Autodesk Inventor part; units mm, degrees
ref_plane "YZ Plane" through (0, 0, 0) normal (1, 0, 0) x (0, 1, 0)
ref_plane "XZ Plane" through (0, 0, 0) normal (0, 1, 0) x (-1, 0, 0)
ref_plane "XY Plane" through (0, 0, 0) normal (0, 0, 1) x (1, 0, 0)
sketch "Sketch1" plane through (0, 0, 0) normal (1, 0, 0) x (0, 1, 0)
  circle A0 centre (0, 0) radius 152.4
  line L0 (-76.2507, 131.953) -> (76.2507, 131.953)
  line L1 (76.2507, 131.953) -> (76.2507, -131.953)
  line L2 (76.2507, -131.953) -> (-76.2507, -131.953)
  line L3 (-76.2507, -131.953) -> (-76.2507, 131.953)
  line L4 (-76.2507, 131.953) -> (76.2507, -131.953) construction
  line L5 (76.2507, 131.953) -> (-76.2507, -131.953) construction
  line L6 (-76.2507, 131.953) -> (-88.9591, 153.9452)
  line L7 (-76.2507, -131.953) -> (-88.9591, -153.9452)
  arc A1 (-88.9591, 153.9452) -> (-88.9591, -153.9452) centre (0, 0) ccw
  line L8 (-88.9591, 153.9452) -> (-177.8, 153.9452)
  line L9 (-177.8, 153.9452) -> (-177.8, -354.0548)
  line L10 (-177.8, -354.0548) -> (0, -354.0548)
  line L11 (0, -354.0548) -> (0, -430.2548)
  line L12 (0, -430.2548) -> (-127, -430.2548)
  line L13 (-127, -430.2548) -> (-127, -354.0548)
  line L14 (-127, -430.2548) -> (-177.8, -430.2548)
  line L15 (-177.8, -430.2548) -> (-177.8, -354.0548)
  line L16 (0, -354.0548) -> (12.7, -354.0548)
  line L17 (12.7, -354.0548) -> (-150.4905, -94.6861)
  line L18 (12.7, -354.0548) -> (34.1986, -340.5282)
  line L19 (34.1986, -340.5282) -> (-128.9918, -81.1595)
  line L20 (12.7, -354.0548) -> (60.6438, -430.2548)
  line L21 (60.6438, -430.2548) -> (82.1424, -416.7282)
  line L22 (82.1424, -416.7282) -> (34.1986, -340.5282)
  line L23 (-177.8, 0) -> (127, 0)
  circle A2 centre (127, 0) radius 304.8
  line L24 (-82.6049, 142.9491) -> (-121.1364, 92.4756)
  line L25 (0, -430.2548) -> (0, -455.6548)
  line L26 (0, -455.6548) -> (235.9429, -455.6548)
  line L27 (82.1424, -416.7282) -> (106.6344, -455.6548)
  line L28 (106.6344, -455.6548) -> (85.1357, -469.1814)
  line L29 (85.1357, -469.1814) -> (60.6438, -430.2548)
  line L30 (95.885, -462.4181) -> (91.6297, -455.6548)
  line L31 (91.6297, -455.6548) -> (98.393, -466.4042)
  line L32 (98.393, -466.4042) -> (120.7006, -452.3686)
  line L33 (106.6344, -455.6548) -> (109.1423, -459.6409)
  line L34 (98.393, -466.4042) -> (67.8539, -485.6188)
  line L35 (85.1357, -469.1814) -> (87.6437, -473.1674)
  line L36 (109.1423, -459.6409) -> (87.6437, -473.1674)
  arc A3 (-88.9591, 153.9452) -> (-150.4905, -94.6861) centre (0, 0) ccw
  line L37 (-128.9918, -81.1595) -> (109.1423, -459.6409)
  line L38 (-150.4905, -94.6861) -> (87.6437, -473.1674)
  line L39 (87.6437, -473.1674) -> (109.1423, -459.6409)
  dimension "d5" = 304.8
  dimension "d6" = 263.906
  dimension "d7" = 25.4
  dimension "d8" = 25.4
  dimension "d9" = 508
  dimension "d10" = 76.2
  dimension "d11" = 127
  dimension "d12" = 12.7
  dimension "d13" = 25.4
  dimension "d14" = 25.4
  dimension "d15" = 304.8
  dimension "d16" = 25.4
  dimension "d17" = 12.7
extrude "Extrusion1" add sketch "Sketch1" along normal blind 6.35 contours A0 L23 A1 L6 L24 | L19 L7 A1 L23 A0 | L19 A2 L17 A1 L7 | L19 L18 L17 A2 | L22 L21 L20 L18 | L27 L26 L29 L21 | L28 L30 L26 | L33 L32 L31 L28 | L26 L30 L28 L29 | L31 L34 L35 L28
sketch "Sketch2" plane through (6.35, 0, 0) normal (1, 0, 0) x (0, 0, -1)
  line L0 (473.1674, 87.6437) -> (459.6409, 109.1423)
  line L1 (-142.9491, -82.6049) -> (-153.9452, -88.9591)
  line L2 (466.4042, 98.393) -> (455.4081, 92.0388)
  circle A0 centre (455.4081, 92.0388) radius 3.175
  dimension "d20" = 12.7
  dimension "d21" = 6.35
extrude "Extrusion2" cut sketch "Sketch2" against normal blind 25.4
sketch "Sketch3" plane through (6.35, 109.1423, -459.6409) normal (0, 0.5325427, -0.8464031) x (-1, 0, 0)
  line L0 (6.35, -25.4) -> (6.35, 0)
  line L1 (6.35, 0) -> (0, 0)
  line L2 (0, -25.4) -> (0, 0)
  line L3 (6.35, -25.4) -> (0, -25.4)
  point P0 (6.35, 152.4)
extrude "Extrusion3" add sketch "Sketch3" along normal blind 508
properties part number "MammothTusk"
Can you work these out from the model? Positions are in its coordinate system, mm. Round coordinates to 2 decimals unless told otherwise and drop trailing zeros. Loops run counter-clockwise (first coordinate to the right, second up) from the corner with the lowest first, then second, coordinate; pieces in that order, holes last. Notation, with made-up numbers: (28, -28.75) -> (86, -28.75) arc R32 ccw to (86, 5.25) -> close; hole circle Ø4 at (7.5, -1). An arc over 180 degrees is marked (long way). One line per item, written item: value. Start each with the question number.
1. If we section it at A-A, the plane y = -107.5: Write out the boundary of the cut face in (x, z), then the cut area to 3 significant figures.
2. If I drill on probe 1 along Y at (x, z) = (4, 8); probe 2 along Y at (x, z) = (4.5, -455.5); probe 3 along Y at (x, z) = (3.25, 78), over which ranges is the centre line in solid material (lowest first)?
3. If we mould it in two halves opening along Z, with no side actions, what happens to faces 1 (the flat face through (6.35, 53, -373)), 2 (the cylindrical face through (3.131, -152.297, 5.594)), 3 (the flat face through (3.13, -101.6, 118.07)), 4 (the cylindrical face through (3.131, -173.063, 40.768))? For each: pulls with the +Z half, pulls with the -Z half, needs draft (parallel to the pull), parting line crosses it, or undercut.
4. If we section it at C-C, the plane z = -717.5: Write out the boundary of the cut face in (x, y), then the cut area to 3 significant figures.
5. If we section it at D-D, the plane y = -7.5: Write out the boundary of the cut face in (x, z).
6. For pin 1 (1.5 mm diameter, centred on x = 5, y = -55, fed in from +Z); pin 2 (1 mm diameter, centred on x = 5, z = -72, fed in from -Y); pin 3 (10 mm diameter, centred on y = 152.5, z = -527.5, fed in from -X); pin 4 (1.5 mm diameter, centred on x = 3, y = 314, fed in from -Z), each with a flat end and sliding along its axis, tell me the tip position at first contact or that it passes through.
Calculated:
1. outline: (0, -163.01) -> (6.35, -163.01) -> (6.35, -115.32) -> (0, -115.32) -> close; (0, 110.34) -> (6.35, 110.34) -> (6.35, 141.62) -> (0, 141.62) -> close
1. area: 502 mm²
2. probe 1: y = -177.62 to -152.19
2. probe 2: y = 76.53 to 88.87, 95.21 to 106.54
2. probe 3: y = -159.78 to -130.93
3. face 1: needs draft
3. face 2: undercut
3. face 3: undercut
3. face 4: parting line crosses it
4. outline: (0, 241.37) -> (6.35, 241.37) -> (6.35, 271.38) -> (0, 271.38) -> close
4. area: 191 mm²
5. outline: (0, -321.95) -> (6.35, -321.95) -> (6.35, -274.25) -> (0, -274.25) -> close
6. pin 1: stops at z = -197.57
6. pin 2: stops at y = -162.79
6. pin 3: stops at x = 0
6. pin 4: stops at z = -834.12
